Drawing for the job (mm, zero at the part's lowest x, y, z). Give positions to 0.01 mm unless a question says otherwise; leave off trailing zeros. Loops run counter-clockwise (first coordinate to the right, second up) from the corner with the lowest first, then second, coordinate; pieces in that order, holes last. Notation, with made-up numbers: M -31,53.5 L 5,53.5 A21 ccw 5,68.5 Z; hole C 52.5,70.5 d11. An arc over 180 degrees is marked long. Answer in a Markdown table with one row per item. Add a question column.
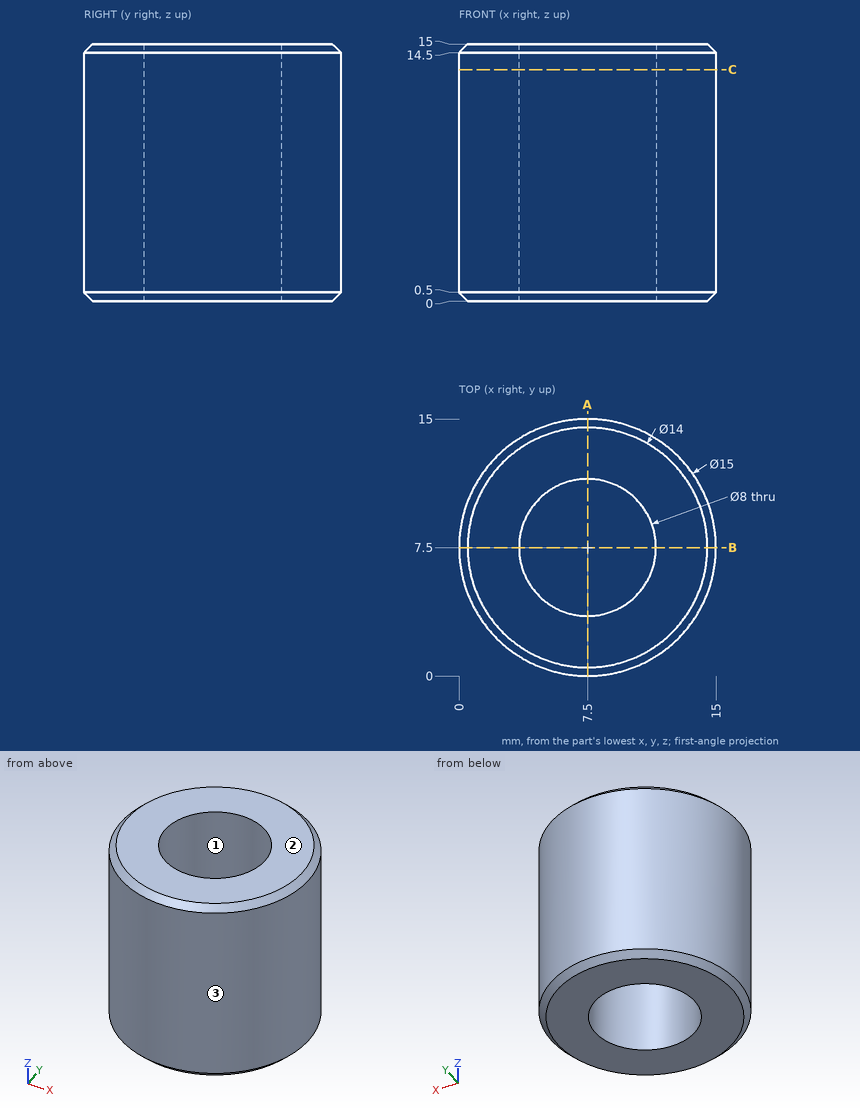
(1) Slice it at C-C, the plane z = 13.5. Give the cut face in (x, y), then the cut area to 3 significant figures.
(2) Pin check, flat tips, straight feed: pin 1 (3 mm diameter, centred on x = 7, y = 7.5, fed in from +Z); pin 2 (2 mm diameter, centred on x = 2, z = 6.5, fed in from -Y). Stop position of each tip, or through.
(3) Wall check: line 1 (Y direction, x = 7.5, z = 8.5); line 2 (X direction, y = 9, z = 12.5). Give the ranges that are in metal, low to high.
(4) Pull direction Y, two halves, no side cores. Call the marked faces 1, 2 and 3: +Y half, -Y half, draft (parallel to the pull), parting line (faces both ways), or undercut.
(5) Slice it at A-A, the plane x = 7.5. Give the cut face in (y, z), then the cut area to 4 significant figures.
Solution:
| question | item | result |
|---|---|---|
| 1 | outline | C 7.5,7.5 d15; hole C 7.5,7.5 d8 |
| 1 | area | 126 mm^2 |
| 2 | pin 1 | through |
| 2 | pin 2 | y = 1.5 |
| 3 | line 1 | 0 to 3.5, 11.5 to 15 |
| 3 | line 2 | 0.15 to 3.79, 11.21 to 14.85 |
| 4 | face 1 | undercut |
| 4 | face 2 | draft |
| 4 | face 3 | parting line |
| 5 | outline | M 0,0.5 L 0.5,0 L 3.5,0 L 3.5,15 L 0.5,15 L 0,14.5 Z; M 11.5,0 L 14.5,0 L 15,0.5 L 15,14.5 L 14.5,15 L 11.5,15 Z |
| 5 | area | 104.5 mm^2 |
